```python
from build123d import *

# Parameters (mm, degrees)
SKETCH1_W                      = 50
SKETCH1_H                      = 75
BOSS_EXTRUDE1_DEPTH            = 3
SKETCH2_W                      = 50
SKETCH2_H                      = 3
BOSS_EXTRUDE2_DEPTH            = 20
M5_CLEARANCE_HOLE1_D           = 5.5
M5_CLEARANCE_HOLE1_ON_FACE_2_D = 5.5
SKETCH6_R                      = 1.5
BOSS_EXTRUDE3_DEPTH            = 2
CUT_EXTRUDE1_REACH             = 50.531
SKETCH7_R                      = 0.6
FILLET1_R                      = 2


with BuildPart() as part:
    # Sketch1 → Boss-Extrude1 (new body)
    with BuildSketch(Plane(origin=(0, 0, 0), x_dir=(1, 0, 0), z_dir=(0, 1, 0))):
        Rectangle(SKETCH1_W, SKETCH1_H)
    extrude(amount=BOSS_EXTRUDE1_DEPTH)

    # Sketch2 → Boss-Extrude2 (add)
    with BuildSketch(Plane(origin=(0, 3, 0), x_dir=(1, 0, 0), z_dir=(0, 1, 0))):
        with Locations((0, 36)):
            Rectangle(SKETCH2_W, SKETCH2_H)
    extrude(amount=BOSS_EXTRUDE2_DEPTH)

    # M5 Clearance Hole1 (through all)
    with Locations(Plane(origin=(20, 11.5, -37.5), x_dir=(-1, 0, 0), z_dir=(0, 0, -1))):
        with Locations((0, 0), (40, 0)):
            Hole(M5_CLEARANCE_HOLE1_D / 2)

    # M5 Clearance Hole1 on face 2 (through all)
    with Locations(Plane(origin=(-94.663434395, 64.222873605, 0), x_dir=(-1, 0, 0), z_dir=(0, 0, -1))):
        with Locations((0, 0)):
            Hole(M5_CLEARANCE_HOLE1_ON_FACE_2_D / 2)

    # Sketch6 → Boss-Extrude3 (add)
    with BuildSketch(Plane(origin=(0, 3, 0), x_dir=(1, 0, 0), z_dir=(0, 1, 0))):
        with Locations(Location((-12.5, 31, 0), (0, 0, 270))):
            Circle(SKETCH6_R)
        with Locations(Location((12.5, 31, 0), (0, 0, 270))):
            Circle(SKETCH6_R)
        with Locations(Location((12.5, -34, 0), (0, 0, 270))):
            Circle(SKETCH6_R)
        with Locations(Location((-12.5, -34, 0), (0, 0, 270))):
            Circle(SKETCH6_R)
    extrude(amount=BOSS_EXTRUDE3_DEPTH)

    # Sketch7 → Cut-Extrude1 (cut, up to next)
    with BuildSketch(Plane(origin=(0, 5, 0), x_dir=(1, 0, 0), z_dir=(0, 1, 0)), mode=Mode.PRIVATE) as cut_extrude1_sk1:
        with Locations(Location((-12.5, 31, 0), (0, 0, 270))):
            Circle(SKETCH7_R)
    cut_extrude1_tool1 = extrude(cut_extrude1_sk1.sketch, amount=-CUT_EXTRUDE1_REACH, mode=Mode.PRIVATE) & part.part
    # Sketch7 → Cut-Extrude1 (cut, up to next)
    with BuildSketch(Plane(origin=(0, 5, 0), x_dir=(1, 0, 0), z_dir=(0, 1, 0)), mode=Mode.PRIVATE) as cut_extrude1_sk2:
        with Locations(Location((12.5, 31, 0), (0, 0, 270))):
            Circle(SKETCH7_R)
    cut_extrude1_tool2 = extrude(cut_extrude1_sk2.sketch, amount=-CUT_EXTRUDE1_REACH, mode=Mode.PRIVATE) & part.part
    # Sketch7 → Cut-Extrude1 (cut, up to next)
    with BuildSketch(Plane(origin=(0, 5, 0), x_dir=(1, 0, 0), z_dir=(0, 1, 0)), mode=Mode.PRIVATE) as cut_extrude1_sk3:
        with Locations(Location((12.5, -34, 0), (0, 0, 270))):
            Circle(SKETCH7_R)
    cut_extrude1_tool3 = extrude(cut_extrude1_sk3.sketch, amount=-CUT_EXTRUDE1_REACH, mode=Mode.PRIVATE) & part.part
    # Sketch7 → Cut-Extrude1 (cut, up to next)
    with BuildSketch(Plane(origin=(0, 5, 0), x_dir=(1, 0, 0), z_dir=(0, 1, 0)), mode=Mode.PRIVATE) as cut_extrude1_sk4:
        with Locations(Location((-12.5, -34, 0), (0, 0, 270))):
            Circle(SKETCH7_R)
    cut_extrude1_tool4 = extrude(cut_extrude1_sk4.sketch, amount=-CUT_EXTRUDE1_REACH, mode=Mode.PRIVATE) & part.part
    add(cut_extrude1_tool1.solids().sort_by_distance((-12.5, 5, -31))[0], mode=Mode.SUBTRACT)
    add(cut_extrude1_tool2.solids().sort_by_distance((12.5, 5, -31))[0], mode=Mode.SUBTRACT)
    add(cut_extrude1_tool3.solids().sort_by_distance((12.5, 5, 34))[0], mode=Mode.SUBTRACT)
    add(cut_extrude1_tool4.solids().sort_by_distance((-12.5, 5, 34))[0], mode=Mode.SUBTRACT)

    # Fillet1
    fillet1_edges = [part.edges().sort_by_distance(p)[0] for p in [
        (-12.5, 3, -32.5),
        (12.5, 3, -32.5),
        (12.5, 3, 32.5),
        (-12.5, 3, 32.5),
    ]]
    fillet(fillet1_edges, radius=FILLET1_R - 0.0001)  # a hair under: the kernel refuses the full size


solid = part.part
```
Build history of the part. All positions in model axes, mm. A direction names the side the tool comes from. Round coordinates to 2 decimals unless told otherwise and drop trailing zeros. Loops run counter-clockwise (first coordinate to the right, second up) from the corner with the lowest first, then second, coordinate; pieces in that order, holes last.
Item 1: Saw through at C-C (z = -26). List the corners of the cut face in (x, y).
Item 2: Pin check, flat tips, straight feed: P1, Ø1.1, axis at x = 12.5, z = -31, coming from the -Y side; P2, Ø1, axis at x = 20, z = 6, coming from the +Y side; P3, Ø2.5, axis at x = -12.5, z = -30.5, coming from the +Y side; P4, Ø3, axis at x = -10, y = 8.5, coming from the +Z side. Stop position of each tip, or through.
Item 3: Drill centre lines: line 1 along X through (y, z) = (1.6, -31); line 2 along Y through (x, z) = (20, -36.4); line 3 along Y through (x, z) = (17, 29). Where is each one in solid material? Low to high.
Item 4: Saw through at B-B (y = 11.5). List the corners of the cut face in (x, z).
Item 5: Saw through at A-A (x = -20). List the corners of the cut face in (y, z), then the cut area to 4 significant figures.
Item 6: Which spindle directions (+Z, -Z, +X, -X, +Y, -Y) get a long thin tool onto all of the face, cutting with end or side? Do faces 4 (the face through (0, 0, -1)), 5 (the face through (0, 3, 1)), 6 (the face through (13, 5, 35)). Say none if no direction does.
Item 7: Two-plate mould, pull along X, no slides. Class faces 1 (the face through (0, 13, -34.5)), 2 (the face through (-25, 2, -5)), 3 (the face through (-22.747, 11.621, -35.979)): released by +X, released by -X, zero draft, split by the parting line, or undercut.
Item 8: Saw through at D-D (x = 2). List the corners of the cut face in (y, z), then the cut area to 3 significant figures.
Worked answers:
1. outline: (-25, 0) - (25, 0) - (25, 3) - (-25, 3) - close
2. P1: passes through
2. P2: stops at y = 3
2. P3: stops at y = 5
2. P4: stops at z = -34.5
3. line 1: x = -25 to -13.1, -11.9 to 11.9, 13.1 to 25
3. line 2: y = 0 to 8.75, 14.25 to 23
3. line 3: y = 0 to 3
4. outline: (-25, -37.5) - (-22.75, -37.5) - (-22.75, -34.5) - (-25, -34.5) - close; (-17.25, -37.5) - (17.25, -37.5) - (17.25, -34.5) - (-17.25, -34.5) - close; (22.75, -37.5) - (25, -37.5) - (25, -34.5) - (22.75, -34.5) - close
5. outline: (0, -37.5) - (8.75, -37.5) - (8.75, -34.5) - (3, -34.5) - (3, 37.5) - (0, 37.5) - close; (14.25, -37.5) - (23, -37.5) - (23, -34.5) - (14.25, -34.5) - close
5. area: 268.5 mm2
6. face 4: +Z, -Z, +X, -X, -Y
6. face 5: +Y
6. face 6: +Z, +X, -X, +Y
7. face 1: zero draft
7. face 2: released by -X
7. face 3: undercut
8. outline: (0, -37.5) - (23, -37.5) - (23, -34.5) - (3, -34.5) - (3, 37.5) - (0, 37.5) - close
8. area: 285 mm2
